```python
from build123d import *

# Parameters (mm, degrees)
F0_R     = 76.4311452349
F0_R_2   = 65
F1_DEPTH = 100
F0_W     = 170
F0_H     = 170
F2_DEPTH = 7
F3_W     = 170
F3_H     = 170
F4_DEPTH = 5
F6_DEPTH = 22.7544467966


with BuildPart() as f1:
    # F0 (on Top) → F1 (new body)
    with BuildSketch(Plane.XY):
        Circle(F0_R)
        Circle(F0_R_2, mode=Mode.SUBTRACT)
    extrude(amount=-F1_DEPTH)

    # F0 (on Top) → F2 (join)
    with BuildSketch(Plane.XY):
        Rectangle(F0_W, F0_H)
        Circle(F0_R, mode=Mode.SUBTRACT)
    extrude(amount=-F2_DEPTH)

    # F3 (on face) → F4 (join)
    with BuildSketch(Plane(origin=(0, 0, -100), x_dir=(1, 0, 0), z_dir=(0, 0, -1))):
        Rectangle(F3_W, F3_H)
    extrude(amount=F4_DEPTH)

    # F5 (on face) → F6 (cut, up to face)
    with BuildSketch(Plane.YZ.offset(85)):
        Polygon((-15, -100), (15, -100), (15, -70), (0, -70), (-15, -70), align=None)
    extrude(amount=-F6_DEPTH, mode=Mode.SUBTRACT)


solid = f1.part
```
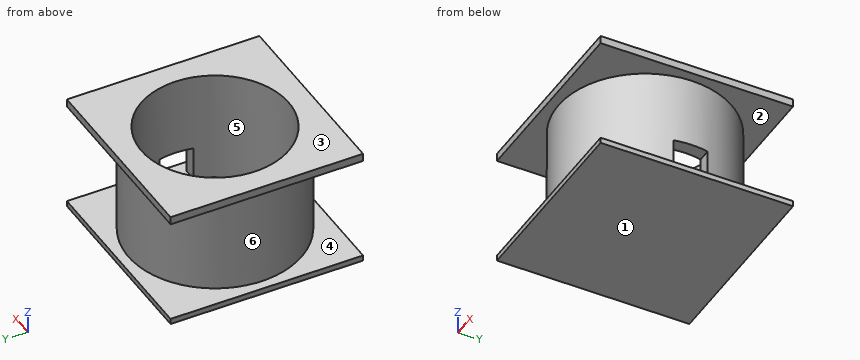
Here's how the part is built. I have some questions about the finished solid (model axes, mm). Face numbers are marked on the shaded views. A direction names the side the tool comes from. Coordinates: 2 decimals unless noted, no trailing zeros. Order: outer loops, then holes, each group sorted by start corner. A loop starts at its lowest first (then second) coordinate and runs counter-clockwise, first axis right, second up.
Item 1: I need wall thicknesses on probe 1 along Z at (x, y) = (-59.5, -61); probe 2 along X at (y, z) = (1, -60); probe 3 along Y at (x, z) = (0, -66). Which ranges of each line are inside material? Lowest first, please.
Response values:
probe 1: z = -105 to -100, -7 to 0
probe 2: x = -76.42 to -64.99, 64.99 to 76.42
probe 3: y = -76.43 to -65, 65 to 76.43
Item 2: If we section it at D-D, the plane y = 22: List the corners of the cut face in (x, z) for me.
Response values:
outline: (-85, -105) - (85, -105) - (85, -100) - (73.2, -100) - (73.2, -7) - (85, -7) - (85, 0) - (61.16, 0) - (61.16, -100) - (-61.16, -100) - (-61.16, 0) - (-85, 0) - (-85, -7) - (-73.2, -7) - (-73.2, -100) - (-85, -100) - close
Item 3: If we section it at B-B, the plane x = 0: List the corners of the cut face in (y, z) for me, then the cut area to 3 significant figures.
Response values:
outline: (-85, -105) - (85, -105) - (85, -100) - (76.43, -100) - (76.43, -7) - (85, -7) - (85, 0) - (65, 0) - (65, -100) - (-65, -100) - (-65, 0) - (-85, 0) - (-85, -7) - (-76.43, -7) - (-76.43, -100) - (-85, -100) - close
area: 3,260 mm2
Item 4: Which directions (+Z, -Z, +X, -X, +Y, -Y) give clear straight access to the entire face, cutting with the end or side of a thin tool? Please do the marked faces 5 and 6.
Response values:
face 5: +Z
face 6: none
Item 5: If we section it at A-A, the plane y = 0: List the corners of the cut face in (x, z) for me.
Response values:
outline: (-85, -105) - (85, -105) - (85, -100) - (-65, -100) - (-65, 0) - (-85, 0) - (-85, -7) - (-76.43, -7) - (-76.43, -100) - (-85, -100) - close; (65, -70) - (76.43, -70) - (76.43, -7) - (85, -7) - (85, 0) - (65, 0) - close
Item 6: Thinking about a two-plate mould opening in Z: for the marked faces 1, 2, 3 and 4, which applies, pulls with the +Z half, pulls with the -Z half, needs draft (parallel to the pull), parting line crosses it, or undercut?
Response values:
face 1: pulls with the -Z half
face 2: undercut
face 3: pulls with the +Z half
face 4: undercut
Item 7: I'm going to push flat-ended pins straight in: pin 1 Ø4 at (x, z) = (-13.5, -22.5) entering from -Y; pin 2 Ø13 at (x, z) = (69.5, -78.5) entering from -Y; pin 3 Ø4 at (y, z) = (-64.5, -88.5) entering from +X. Where does each tip first touch, or does it pass through?
Response values:
pin 1: stops at y = -75.56
pin 2: stops at y = -43.27
pin 3: stops at x = 43.99
Item 8: If we section it at C-C, the plane z = -95: List the corners of the cut face in (x, y) for me, then the cut area to 3 significant figures.
Response values:
outline: (63.25, -15) arc R65 cw (long way) to (63.25, 15) - (74.94, 15) arc R76.43 ccw (long way) to (74.94, -15) - close
area: 4,730 mm2
